Geometry check sheet. Reference: the model listing, model coordinates, mm. Face numbers are marked on the shaded views. A direction names the side the tool comes from. Give positions to 0.01 mm unless a question says otherwise; leave off trailing zeros. Order: outer loops, then holes, each group sorted by start corner. A loop starts at its lowest first (then second) coordinate and runs counter-clockwise, first axis right, second up.
from build123d import *

# Parameters (mm, degrees)
SKETCH1_W          = 10
SKETCH1_H          = 14.057527786
SKETCH1_R          = 2.287307526
BASE_FLANGE1_DEPTH = 1
EDGE_FLANGE1_DEPTH = 10
EDGE_FLANGE2_DEPTH = 10
SKETCH12_R         = 1.5
CUT_EXTRUDE1_DEPTH = 2
FILLET1_R          = 3


# Sheet-metal steps are written as plain solids
with BuildPart() as part:
    # Sketch1 → Base-Flange1 (new body)
    with BuildSketch(Plane.XY):
        with Locations((-509.974194853, -21.379047402)):
            Rectangle(SKETCH1_W, SKETCH1_H)
        with Locations((-509.974194853, -19.4)):
            Circle(SKETCH1_R, mode=Mode.SUBTRACT)
    extrude(amount=BASE_FLANGE1_DEPTH)

    # Edge-Flange1 section (across the edge) → Edge-Flange1 (add)
    with BuildSketch(Plane(origin=(-514.974194853, -29.144411295, 1), x_dir=(0, 1, 0), z_dir=(1, 0, 0))):
        with BuildLine():
            Line((-1, 0.7366), (-1, 1))
            Line((-1, 1), (0, 1))
            Line((0, 1), (0, 0.7366))
            ThreePointArc((0, 0.7366), (0.215745145, 0.215745145), (0.7366, 0))
            Line((0.7366, 0), (0.7366, -1))
            ThreePointArc((0.7366, -1), (-0.491361636, -0.491361636), (-1, 0.7366))
        make_face()
    extrude(amount=EDGE_FLANGE1_DEPTH)

    # Edge-Flange2 section (across the edge) → Edge-Flange2 (add)
    with BuildSketch(Plane(origin=(-504.974194853, -30.144411295, 2.7366), x_dir=(0, 0, -1), z_dir=(-1, 0, 0))):
        with BuildLine():
            Line((-1, 0.7366), (-1, 10.7366))
            Line((-1, 10.7366), (0, 10.7366))
            Line((0, 10.7366), (0, 0.7366))
            ThreePointArc((0, 0.7366), (0.215745145, 0.215745145), (0.7366, 0))
            Line((0.7366, 0), (0.7366, -1))
            ThreePointArc((0.7366, -1), (-0.491361636, -0.491361636), (-1, 0.7366))
        make_face()
    extrude(amount=EDGE_FLANGE2_DEPTH)

    # Sketch12 → Cut-Extrude1 (cut)
    with BuildSketch(Plane(origin=(0, 0, 2.7366), x_dir=(-1, 0, 0), z_dir=(0, 0, -1))):
        with Locations((509.974194853, -35.881011295)):
            Circle(SKETCH12_R)
    extrude(amount=-CUT_EXTRUDE1_DEPTH, mode=Mode.SUBTRACT)

    # Fillet1
    fillet1_edges = [part.edges().sort_by_distance(p)[0] for p in [
        (-504.974194853, -40.881011295, 3.2366),
        (-514.974194853, -40.881011295, 3.2366),
        (-514.974194853, -14.350283509, 0.5),
        (-504.974194853, -14.350283509, 0.5),
    ]]
    fillet(fillet1_edges, radius=FILLET1_R)


solid = part.part
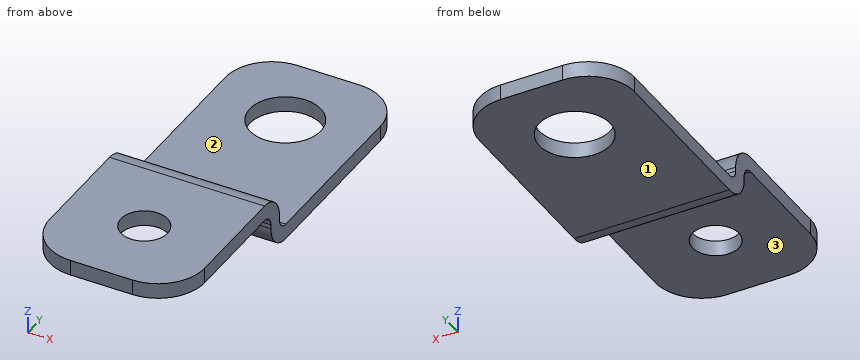
Item 1: Gauge pin test, flat end, axial feed: pin 1 (2.5 mm diameter, centred on x = -509.97, y = -35.88, fed in from -Z). Record the tip position at first contact, or that the pin passes through.
Reported:
pin 1: passes through
Item 2: Set-up check for the marked faces 1, 2 and 3: record each of +Z, -Z, +X, -X, +Y, -Y from which the full face is reachable in a straight line by a thin tool's end or side.
Reported:
face 1: -Z, +X, -X, +Y, -Y
face 2: +Z, +X, -X, +Y
face 3: -Z, +X, -X, -Y
Item 3: Sectioned sample at B-B (z = 0.5). Enter the section's corners in (x, y), and give its area (3 significant figures).
Reported:
outline: (-514.97, -29.63) - (-504.97, -29.63) - (-504.97, -17.35) arc R3 ccw to (-507.97, -14.35) - (-511.97, -14.35) arc R3 ccw to (-514.97, -17.35) - close; hole circle Ø4.57 at (-509.97, -19.4)
area: 132 mm2
Item 4: Scan lines: L1, parallel to Z at x = -507, y = -26.25; L2, parallel to Y at x = -509.25, z = 2.95; L3, parallel to Y at x = -508.25, z = 1.9. Record each from-to range of solid material in increasing order.
Reported:
L1: z = 0 to 1
L2: y = -40.88 to -37.19, -34.57 to -29.43
L3: y = -30.14 to -29.14
Item 5: Sectioned sample at D-D (y = -33). Enter the section's corners in (x, z).
Reported:
outline: (-514.97, 2.74) - (-504.97, 2.74) - (-504.97, 3.74) - (-514.97, 3.74) - close
Item 6: Sectioned sample at A-A (y = -19.4). Enter the section's corners in (x, z).
Reported:
outline: (-514.97, 0) - (-512.26, 0) - (-512.26, 1) - (-514.97, 1) - close; (-507.69, 0) - (-504.97, 0) - (-504.97, 1) - (-507.69, 1) - close
Item 7: Sectioned sample at C-C (x = -514). Enter the section's corners in (y, z).
Reported:
outline: (-40.09, 2.74) - (-30.88, 2.74) arc R0.74 cw to (-30.14, 2) - (-30.14, 1.74) arc R1.74 ccw to (-28.41, 0) - (-15.14, 0) - (-15.14, 1) - (-28.41, 1) arc R0.74 cw to (-29.14, 1.74) - (-29.14, 2) arc R1.74 ccw to (-30.88, 3.74) - (-40.09, 3.74) - close
